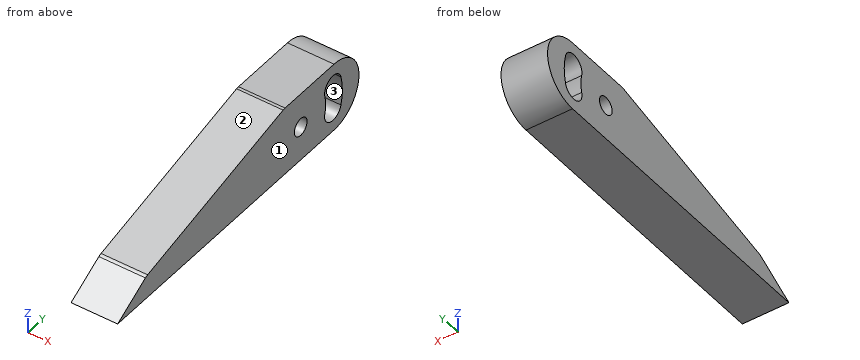
```python
from build123d import *

# Parameters (mm, degrees)
F1_DEPTH = 12.7
F2_D     = 4.826
F3_R     = 3.175


with BuildPart() as f1:
    # F0 (on Right) → F1 (new body)
    with BuildSketch(Plane.YZ):
        with BuildLine():
            Line((10.9985226281, 6.35), (0, 0))
            Line((0, 0), (82.55, 0))
            ThreePointArc((82.55, 0), (92.075, 9.525), (82.55, 19.05))
            Line((82.55, 19.05), (63.5, 19.05))
            Line((63.5, 19.05), (10.9985226281, 6.35))
        make_face()
        with BuildLine():
            ThreePointArc((79.0569245722, 11.9659352556), (81.3122543444, 15.8485551982), (85.194874287, 13.5932254261))
            ThreePointArc((85.194874287, 13.5932254261), (85.725, 9.525), (85.194874287, 5.4567745739))
            ThreePointArc((85.194874287, 5.4567745739), (81.3122543444, 3.2014448018), (79.0569245722, 7.0840647444))
            ThreePointArc((79.0569245722, 7.0840647444), (79.375, 9.525), (79.0569245722, 11.9659352556))
        make_face(mode=Mode.SUBTRACT)
    extrude(amount=F1_DEPTH)

    # F2 (through all)
    with Locations(Plane(origin=(0, 0, 0), x_dir=(0, 1, 0), z_dir=(-1, 0, 0))):
        with Locations((69.85, -9.525), (82.4664258806, -8.070421711)):
            Hole(F2_D / 2)

    # F3
    f3_edges = [f1.edges().sort_by_distance(p)[0] for p in [
        (6.35, 63.5, 19.05),
        (6.35, 10.998523, 6.35),
    ]]
    fillet(f3_edges, radius=F3_R)


solid = f1.part
```
Check sheet for the modelled part. Datum: model origin and axes. Units: mm. Face numbers are marked on the shaded views. Give positions to 0.01 mm unless a question says otherwise; leave off trailing zeros. Loops run counter-clockwise (first coordinate to the right, second up) from the corner with the lowest first, then second, coordinate; pieces in that order, holes last. Notation, with made-up numbers: (65.5, 30) - (74.5, 30) arc R26 cw to (74.5, 50) - close; hole circle Ø11 at (74.5, 52.5). An arc over 180 degrees is marked (long way). One line per question, with ' | ' between items. Start each with the question number.
1. Cross-section at A-A, the plane y = 69.85. Enter the section's corners in (x, z), plus the area to 3 significant figures.
2. Cross-section at D-D, the plane z = 1.5. Enter the section's corners in (x, y).
3. Gauge pin test, flat ends, axial feed: pin 1 Ø5 at (y, z) = (36.5, 13.5) entering from +X; pin 2 Ø5 at (x, y) = (4, 53.5) entering from +Z; pin 3 Ø4 at (x, z) = (8.5, 16.5) entering from +Y. Record the tip position at first contact, or that the pin passes through.
4. Cross-section at B-B, the plane x = 10.75. Enter the section's corners in (y, z) (3 decimals).
5. Cross-section at C-C, the plane y = 81.5. Enter the section's corners in (x, z).
6. Material ranges on line 1 along Z through (x, y) = (3.5, 69.85); line 2 along Y through (x, z) = (9.25, 5.5); line 3 along Z through (x, y) = (2, 84.5), recorded low to high. Write a range as [from, to].
7. Draft check along Z on the marked faces 1, 2 and 3. Enter one of: released by +Z, released by -Z, zero draft, split by the parting line, or undercut.
Check result:
1) outline: (0, 0) - (12.7, 0) - (12.7, 7.11) - (0, 7.11) - close; (0, 11.94) - (12.7, 11.94) - (12.7, 19.05) - (0, 19.05) - close | area: 181 mm2
2) outline: (0, 2.6) - (12.7, 2.6) - (12.7, 87.68) - (0, 87.68) - close
3) pin 1: stops at x = 12.7 | pin 2: stops at z = 17.24 | pin 3: stops at y = 90.67
4) outline: (0, 0) - (82.55, 0) arc R9.525 ccw to (82.55, 19.05) - (63.879, 19.05) arc R3.175 ccw to (63.132, 18.961) - (11.443, 6.458) arc R3.175 ccw to (10.602, 6.121) - close; hole circle Ø4.826 at (69.85, 9.525); hole (79.057, 7.084) arc R3.175 ccw to (85.195, 5.457) arc R15.875 ccw to (85.195, 13.593) arc R3.175 ccw to (79.057, 11.966) arc R9.525 cw to start
5) outline: (0, 0) - (12.7, 0) - (12.7, 3.16) - (0, 3.16) - close; (0, 15.89) - (12.7, 15.89) - (12.7, 19.05) - (0, 19.05) - close
6) line 1: z = [0, 7.11], [11.94, 19.05] | line 2: y = [9.53, 79.05], [85.21, 91.18] | line 3: z = [0.2, 4.16], [14.89, 18.85]
7) face 1: zero draft | face 2: released by +Z | face 3: undercut
